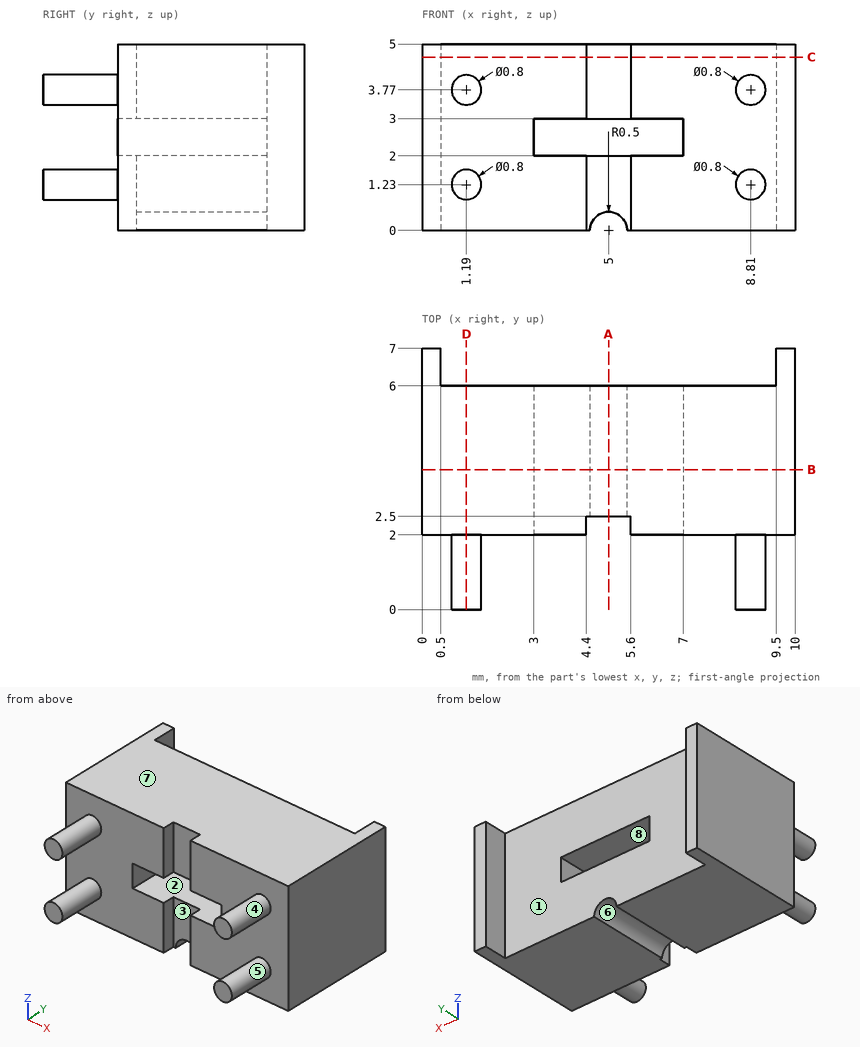
Answer from the drawing. Dimensions are ordinates in mm from the lowest x, y and z of the part. A direction names the side the tool comes from. Round coordinates to 2 decimals unless told otherwise and drop trailing zeros. Order: outer loops, then holes, each group sorted by start corner. A loop starts at its lowest first (then second) coordinate and runs counter-clockwise, first axis right, second up.
1) The part is cut by section B-B on y = 3.75. Write down the section's boundary in (x, z), plus the area to 3 significant figures.
2) The part is cut by section C-C on z = 4.65. Write down the section's boundary in (x, y), plus the area to 3 significant figures.
3) The mould has two halves that part along Z. Classify the marked faces 5, 6, 7 and 8: released by +Z, released by -Z, zero draft, split by the parting line, or undercut.
4) For the marked faces 1, 2, 3 and 4, determine the directions among +Z, -Z, +X, -X, +Y, -Y from which every point of the face is accessible in a straight line to the end or side of a thin tool.
5) The part is cut by section D-D on x = 1.19. Write down the section's boundary in (y, z).
6) Straight lines are drawn through the part: L1, parallel to X at y = 2.25, z = 4.6; L2, parallel to X at y = 2.5, z = 2.65; L3, parallel to Y at x = 2.5, z = 0.9. For each, find the intervals that lie inside material, in ascending order.
7) Flat-ended cylindrical pins translate along their axes: pin 1 (1 mm diameter, centred on x = 4.5, z = 3.5, fed in from -Y); pin 2 (1 mm diameter, centred on x = 6.5, z = 1.5, fed in from +Y). Find the tip coordinate at first contact, or state that the pin passes through.
8) The part is cut by section A-A on x = 5. Write down the section's boundary in (y, z).
Resolved:
1. outline: (0, 0) - (4.5, 0) arc R0.5 cw to (5.5, 0) - (10, 0) - (10, 5) - (0, 5) - close; hole (3, 2) - (7, 2) - (7, 3) - (3, 3) - close
1. area: 45.6 mm2
2. outline: (0, 2) - (4.4, 2) - (4.4, 2.5) - (5.6, 2.5) - (5.6, 2) - (10, 2) - (10, 7) - (9.5, 7) - (9.5, 6) - (0.5, 6) - (0.5, 7) - (0, 7) - close
2. area: 40.4 mm2
3. face 5: undercut
3. face 6: released by -Z
3. face 7: released by +Z
3. face 8: undercut
4. face 1: +Z, -Z, +Y
4. face 2: +Y, -Y
4. face 3: +Z, -Z, -Y
4. face 4: -Y
5. outline: (0, 0.83) - (2, 0.83) - (2, 0) - (6, 0) - (6, 5) - (2, 5) - (2, 4.17) - (0, 4.17) - (0, 3.37) - (2, 3.37) - (2, 1.63) - (0, 1.63) - close
6. L1: x = 0 to 4.4, 5.6 to 10
6. L2: x = 0 to 3, 7 to 10
6. L3: y = 2 to 6
7. pin 1: stops at y = 2
7. pin 2: stops at y = 6
8. outline: (2.5, 0.5) - (6, 0.5) - (6, 2) - (2.5, 2) - close; (2.5, 3) - (6, 3) - (6, 5) - (2.5, 5) - close
